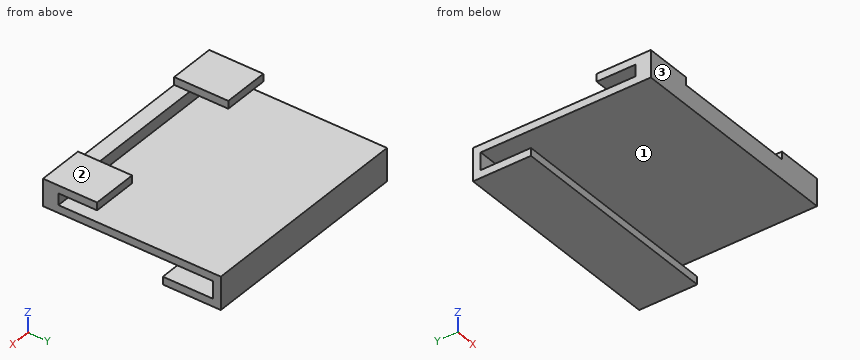
from build123d import *

# Parameters (mm, degrees)
F0_W     = 57
F0_H     = 4
F0_H_2   = 2
F0_H_3   = 40
F1_DEPTH = 2
F2_DEPTH = 3
F3_W     = 12
F3_H     = 14
F4_DEPTH = 2
F5_DEPTH = 6.5
F6_W     = 57
F6_H     = 15
F7_DEPTH = 2


with BuildPart() as f1:
    # F0 (on Top) → F1 (new body)
    with BuildSketch(Plane.XY):
        with Locations((0, -21)):
            Rectangle(F0_W, F0_H)
        with Locations((0, 22)):
            Rectangle(F0_W, F0_H_2)
        with Locations((0, 1)):
            Rectangle(F0_W, F0_H_3)
    extrude(amount=-F1_DEPTH)

    # F0 (on Top) → F2 (join)
    with BuildSketch(Plane.XY):
        with Locations((0, -21)):
            Rectangle(F0_W, F0_H)
    extrude(amount=F2_DEPTH)

    # F3 (on face) → F4 (join)
    with BuildSketch(Plane.XY.offset(3)):
        with Locations((-22.5, -16)):
            Rectangle(F3_W, F3_H)
        with Locations((22.5, -16)):
            Rectangle(F3_W, F3_H)
    extrude(amount=F4_DEPTH)

    # F0 (on Top) → F5 (join)
    with BuildSketch(Plane.XY):
        with Locations((0, 22)):
            Rectangle(F0_W, F0_H_2)
    extrude(amount=-F5_DEPTH)

    # F6 (on face) → F7 (join)
    with BuildSketch(Plane(origin=(0, 0, -6.5), x_dir=(1, 0, 0), z_dir=(0, 0, -1))):
        with Locations((0, -15.5)):
            Rectangle(F6_W, F6_H)
    extrude(amount=F7_DEPTH)


solid = f1.part
Verification items for the finished model (mm, model axes). Face numbers are marked on the shaded views. Round coordinates to 2 decimals unless told otherwise and drop trailing zeros. Write each loop counter-clockwise with the first axis right and the second up, starting at its lowest first coordinate (ties: lowest second). Pieces come first, ordered by that corner, then holes.
(1) Section check C-C (y = -17.5). Enter the section's corners in (x, z).
Returned:
outline: (-28.5, -2) - (28.5, -2) - (28.5, 0) - (-28.5, 0) - close; (-28.5, 3) - (-16.5, 3) - (-16.5, 5) - (-28.5, 5) - close; (16.5, 3) - (28.5, 3) - (28.5, 5) - (16.5, 5) - close
(2) Section check B-B (x = -20.5). Enter the section's corners in (y, z), plus the area to 3 significant figures.
Returned:
outline: (-23, -2) - (21, -2) - (21, -6.5) - (8, -6.5) - (8, -8.5) - (23, -8.5) - (23, 0) - (-19, 0) - (-19, 3) - (-9, 3) - (-9, 5) - (-23, 5) - close
area: 171 mm2
(3) Section check A-A (y = 13.5). Enter the section's corners in (x, z).
Returned:
outline: (-28.5, -8.5) - (28.5, -8.5) - (28.5, -6.5) - (-28.5, -6.5) - close; (-28.5, -2) - (28.5, -2) - (28.5, 0) - (-28.5, 0) - close
(4) Depth check by flat-ended pin: pin 1 Ø12.5 at (x, y) = (13, 8.5) entering from +Z; pin 2 Ø2 at (x, z) = (-10, -7.5) entering from -Y; pin 3 Ø5 at (x, y) = (-25, -14.5) entering from -Z. Enter the tip coordinate at first touch or a pass-through.
Returned:
pin 1: stops at z = 0
pin 2: stops at y = 8
pin 3: stops at z = -2
(5) Material ranges on line 1 (Y direction, x = 20, z = 3.5); line 2 (Z direction, x = -15, y = -2); line 3 (Z direction, x = 26.5, y = -20), recorded low to high.
Returned:
line 1: y = -23 to -9
line 2: z = -2 to 0
line 3: z = -2 to 5
(6) Section check D-D (z = -3.25). Enter the section's corners in (x, y), plus the area to 3 significant figures.
Returned:
outline: (-28.5, 21) - (28.5, 21) - (28.5, 23) - (-28.5, 23) - close
area: 114 mm2
(7) Mould release check, pull along Z, two halves, no side actions. Record for the marked faces 1, 2 and 3: pulls with the +Z half, pulls with the -Z half, needs draft (parallel to the pull), parting line crosses it, or undercut.
Returned:
face 1: undercut
face 2: pulls with the +Z half
face 3: needs draft
